```python
from build123d import *

# Parameters (mm, degrees)
ESQUISSE1_W              = 250
ESQUISSE1_H              = 25
BOSS_EXTRU_1_DEPTH       = 5
ESQUISSE2_W              = 5
ESQUISSE2_H              = 5
ENL_V_MAT_EXTRU_1_DEPTH  = 5
SYM_TRIE1_DEPTH          = 5
ESQUISSE3_W              = 5
ESQUISSE3_H              = 5
ENL_V_MAT_EXTRU_14_DEPTH = 5


# Read off the part's stored shape, not the designer's step: Symétrie1
with BuildPart() as part:
    # Esquisse1 → Boss.-Extru.1 (new body)
    with BuildSketch(Plane.XY):
        with Locations((60.132935366, -9.243939394)):
            Rectangle(ESQUISSE1_W, ESQUISSE1_H)
    extrude(amount=BOSS_EXTRU_1_DEPTH)

    # Esquisse2 → Enlèv. mat.-Extru.1 (cut)
    with BuildSketch(Plane.XY.offset(5)):
        with Locations((177.632935366, 0.756060606)):
            Rectangle(ESQUISSE2_W, ESQUISSE2_H)
        with Locations((167.632935366, 0.756060606)):
            Rectangle(ESQUISSE2_W, ESQUISSE2_H)
        with Locations((-25.367064634, 0.756060606)):
            Rectangle(ESQUISSE2_W, ESQUISSE2_H)
        with Locations((-35.367064634, 0.756060606)):
            Rectangle(ESQUISSE2_W, ESQUISSE2_H)
        with Locations((-52.367064634, 0.756060606)):
            Rectangle(ESQUISSE2_W, ESQUISSE2_H)
        with Locations((-62.367064634, 0.756060606)):
            Rectangle(ESQUISSE2_W, ESQUISSE2_H)
        with Locations((182.632935366, -9.243939394)):
            Rectangle(ESQUISSE2_W, ESQUISSE2_H)
        with Locations((182.632935366, -19.243939394)):
            Rectangle(ESQUISSE2_W, ESQUISSE2_H)
        with BuildLine():
            Line((84.132935366, -21.743939394), (85.132935366, -21.743939394))
            Line((85.132935366, -21.743939394), (86.132935366, -21.743939394))
            ThreePointArc((86.132935366, -21.743939394), (85.132935366, -20.743939394), (84.132935366, -21.743939394))
        make_face()
        with BuildLine():
            Line((94.132935366, -21.743939394), (95.132935366, -21.743939394))
            Line((95.132935366, -21.743939394), (96.132935366, -21.743939394))
            ThreePointArc((96.132935366, -21.743939394), (95.132935366, -20.743939394), (94.132935366, -21.743939394))
        make_face()
    extrude(amount=-ENL_V_MAT_EXTRU_1_DEPTH, mode=Mode.SUBTRACT)

    # Symétrie1 outline → Symétrie1 (add)
    with BuildSketch(Plane.XY):
        with BuildLine():
            Line((180.132935366, -31.743939394), (185.132935366, -31.743939394))
            Line((185.132935366, -31.743939394), (185.132935366, -26.743939394))
            Line((185.132935366, -26.743939394), (180.132935366, -26.743939394))
            Line((180.132935366, -26.743939394), (180.132935366, -21.743939394))
            Line((180.132935366, -21.743939394), (96.132935366, -21.743939394))
            ThreePointArc((96.132935366, -21.743939394), (95.132935366, -22.743939394), (94.132935366, -21.743939394))
            Line((94.132935366, -21.743939394), (86.132935366, -21.743939394))
            ThreePointArc((86.132935366, -21.743939394), (85.132935366, -22.743939394), (84.132935366, -21.743939394))
            Line((84.132935366, -21.743939394), (-64.867064634, -21.743939394))
            Line((-64.867064634, -21.743939394), (-64.867064634, -41.743939394))
            Line((-64.867064634, -41.743939394), (-59.867064634, -41.743939394))
            Line((-59.867064634, -41.743939394), (-59.867064634, -46.743939394))
            Line((-59.867064634, -46.743939394), (-54.867064634, -46.743939394))
            Line((-54.867064634, -46.743939394), (-54.867064634, -41.743939394))
            Line((-54.867064634, -41.743939394), (-49.867064634, -41.743939394))
            Line((-49.867064634, -41.743939394), (-49.867064634, -46.743939394))
            Line((-49.867064634, -46.743939394), (-37.867064634, -46.743939394))
            Line((-37.867064634, -46.743939394), (-37.867064634, -41.743939394))
            Line((-37.867064634, -41.743939394), (-32.867064634, -41.743939394))
            Line((-32.867064634, -41.743939394), (-32.867064634, -46.743939394))
            Line((-32.867064634, -46.743939394), (-27.867064634, -46.743939394))
            Line((-27.867064634, -46.743939394), (-27.867064634, -41.743939394))
            Line((-27.867064634, -41.743939394), (-22.867064634, -41.743939394))
            Line((-22.867064634, -41.743939394), (-22.867064634, -46.743939394))
            Line((-22.867064634, -46.743939394), (165.132935366, -46.743939394))
            Line((165.132935366, -46.743939394), (165.132935366, -41.743939394))
            Line((165.132935366, -41.743939394), (170.132935366, -41.743939394))
            Line((170.132935366, -41.743939394), (170.132935366, -46.743939394))
            Line((170.132935366, -46.743939394), (175.132935366, -46.743939394))
            Line((175.132935366, -46.743939394), (175.132935366, -41.743939394))
            Line((175.132935366, -41.743939394), (180.132935366, -41.743939394))
            Line((180.132935366, -41.743939394), (180.132935366, -46.743939394))
            Line((180.132935366, -46.743939394), (185.132935366, -46.743939394))
            Line((185.132935366, -46.743939394), (185.132935366, -36.743939394))
            Line((185.132935366, -36.743939394), (180.132935366, -36.743939394))
            Line((180.132935366, -36.743939394), (180.132935366, -31.743939394))
        make_face()
    extrude(amount=SYM_TRIE1_DEPTH)

    # Esquisse3 → Enlèv. mat.-Extru.14 (cut)
    with BuildSketch(Plane.XY.offset(5)):
        with Locations((-25.367064634, -4.243939394)):
            Rectangle(ESQUISSE3_W, ESQUISSE3_H)
        with Locations((-25.367064634, -31.743939394)):
            Rectangle(ESQUISSE3_W, ESQUISSE3_H)
    extrude(amount=-ENL_V_MAT_EXTRU_14_DEPTH, mode=Mode.SUBTRACT)


solid = part.part
```
Read the model definition and answer for the solid it produces. Units are mm, in the model's axes. A direction names the side the tool comes from. Give positions to 0.01 mm unless a question says otherwise; leave off trailing zeros. Loops run counter-clockwise (first coordinate to the right, second up) from the corner with the lowest first, then second, coordinate; pieces in that order, holes last.
Item 1: For faces 5 (the flat face through (-25, -6.744, 3)), 6 (the flat face through (168, -41.744, 2)), 7 (the flat face through (-62, -41.744, 2)), 8 (the flat face through (-27.867, -32, 3)), determine the directions among +Z, -Z, +X, -X, +Y, -Y from which every point of the face is accessible in a straight line to the end or side of a thin tool.
Item 2: The mould has two halves that part along X. Classify faces 1 (the flat face through (183, -16.744, 3)), 2 (the flat face through (-59.867, 1, 3)), 3 (the flat face through (180.133, -44, 2)), 4 (the flat face through (168, -1.744, 3)): released by +X, released by -X, zero draft, split by the parting line, or undercut.
Item 3: The part is cut by section A-A (y = -9). Write down the section's boundary in (x, z), and give its area (4 significant figures).
Item 4: Find the intervals of material crossed by line 1 along X through (y, z) = (-21.5, 4.2); line 2 along X through (y, z) = (-43, 2.15); line 3 along Y through (x, z) = (-36.5, 0.95), in increasing order.
Item 5: Each of these flat-tipped pins is pushed along its axis until it touches: pin 1 Ø12 at (x, y) = (76.5, -16) entering from -Z; pin 2 Ø1.5 at (x, z) = (-36.5, 3.5) entering from -Y. Where does it stop, or does it pass through?
Item 6: The part is cut by section B-B (z = 1.25). Give the number of separate pieces and of enclosed holes in the cut face, and give its area (3 significant figures).
Taken from the geometry:
1. face 5: +Z, -Z, +Y
1. face 6: +Z, -Z, -Y
1. face 7: +Z, -Z, -X, -Y
1. face 8: +Z, -Z
2. face 1: zero draft
2. face 2: released by -X
2. face 3: undercut
2. face 4: undercut
3. outline: (-64.87, 0) - (180.13, 0) - (180.13, 5) - (-64.87, 5) - close
3. area: 1,225 mm2
4. line 1: x = -64.87 to 84.16, 86.1 to 94.16, 96.1 to 180.13
4. line 2: x = -59.87 to -54.87, -49.87 to -37.87, -32.87 to -27.87, -22.87 to 165.13, 170.13 to 175.13, 180.13 to 185.13
4. line 3: y = -41.74 to -1.74
5. pin 1: stops at z = 0
5. pin 2: stops at y = -41.74
6. separate pieces: 1
6. enclosed holes: 3
6. area: 12,000 mm2
